Geometry check sheet. Reference: drawing and pictorial views, mm from the part's lowest x, y, z. A direction names the side the tool comes from. Give positions to 0.01 mm unless a question says otherwise; leave off trailing zeros. Write each loop counter-clockwise with the first axis right and the second up, starting at its lowest first coordinate (ties: lowest second). Pieces come first, ordered by that corner, then holes. Notation, with made-up numbers: (6, -18.5) -> (22, -18.5) arc R15 ccw to (22, 10.5) -> close; hole circle Ø11 at (33, 46.5). An arc over 180 degrees is marked (long way). Use a Markdown table: item, result. Add a question column.
1. Cross-section at B-B (z = 6.75). Enter the section's corners in (x, y), then the cut area to 3 significant figures.
2. Scan lines: probe 1 along X at (y, z) = (17.3, 6.25); probe 2 along Y at (x, z) = (8, 11); probe 3 along X at (y, z) = (12.5, 0.75). Record each from-to range of solid material in increasing order. Write a range as [from, to].
3. Gauge pin test, flat ends, axial feed: P1, Ø5, axis at x = 30, z = 6.25, coming from the -Y side; P2, Ø4, axis at y = 9.5, z = 3.5, coming from the -X side; P3, Ø6, axis at y = 9, z = 7.5, coming from the +X side. Record the tip position at first contact, or that the pin passes through.
4. Cross-section at A-A (x = 30). Enter the section's corners in (y, z), then the cut area to 4 significant figures.
5. Cross-section at C-C (x = 22). Enter the section's corners in (y, z), then the cut area to 3 significant figures.
6. Cross-section at D-D (z = 2). Enter the section's corners in (x, y).
7. Release check for a two-part mould opening along Y. For the marked faces 4, 5, 6 and 7 record: released by +Y, released by -Y, zero draft, split by the parting line, or undercut.
8. Set-up check for the marked faces 1, 2 and 3: record each of +Z, -Z, +X, -X, +Y, -Y from which the full face is reachable in a straight line by a thin tool's end or side.
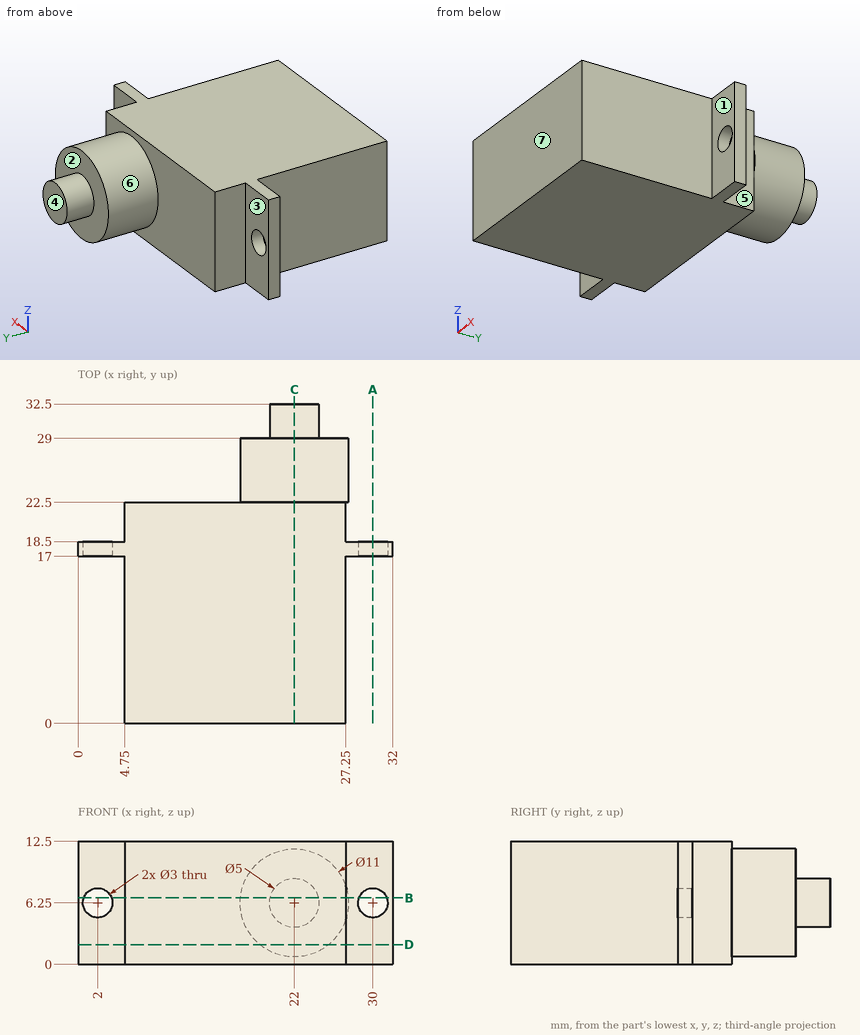
Worked answers:
| question | item | result |
|---|---|---|
| 1 | outline | (0, 17) -> (0.59, 17) -> (0.59, 18.5) -> (0, 18.5) -> close; (3.41, 17) -> (4.75, 17) -> (4.75, 0) -> (27.25, 0) -> (27.25, 17) -> (28.59, 17) -> (28.59, 18.5) -> (27.25, 18.5) -> (27.25, 22.5) -> (27.48, 22.5) -> (27.48, 29) -> (24.45, 29) -> (24.45, 32.5) -> (19.55, 32.5) -> (19.55, 29) -> (16.52, 29) -> (16.52, 22.5) -> (4.75, 22.5) -> (4.75, 18.5) -> (3.41, 18.5) -> close; (31.41, 17) -> (32, 17) -> (32, 18.5) -> (31.41, 18.5) -> close |
| 1 | area | 600 mm² |
| 2 | probe 1 | x = [0, 0.5], [3.5, 28.5], [31.5, 32] |
| 2 | probe 2 | y = [0, 22.5] |
| 2 | probe 3 | x = [4.75, 27.25] |
| 3 | P1 | stops at y = 17 |
| 3 | P2 | stops at x = 4.75 |
| 3 | P3 | stops at x = 27.25 |
| 4 | outline | (17, 0) -> (18.5, 0) -> (18.5, 4.75) -> (17, 4.75) -> close; (17, 7.75) -> (18.5, 7.75) -> (18.5, 12.5) -> (17, 12.5) -> close |
| 4 | area | 14.25 mm² |
| 5 | outline | (0, 0) -> (22.5, 0) -> (22.5, 0.75) -> (29, 0.75) -> (29, 3.75) -> (32.5, 3.75) -> (32.5, 8.75) -> (29, 8.75) -> (29, 11.75) -> (22.5, 11.75) -> (22.5, 12.5) -> (0, 12.5) -> close |
| 5 | area | 370 mm² |
| 6 | outline | (0, 17) -> (4.75, 17) -> (4.75, 0) -> (27.25, 0) -> (27.25, 17) -> (32, 17) -> (32, 18.5) -> (27.25, 18.5) -> (27.25, 22.5) -> (25.49, 22.5) -> (25.49, 29) -> (18.51, 29) -> (18.51, 22.5) -> (4.75, 22.5) -> (4.75, 18.5) -> (0, 18.5) -> close |
| 7 | face 4 | released by +Y |
| 7 | face 5 | undercut |
| 7 | face 6 | zero draft |
| 7 | face 7 | released by -Y |
| 8 | face 1 | +Z, -Z, +X, -Y |
| 8 | face 2 | +Y |
| 8 | face 3 | +Z, -Z, -X, +Y |
